```python
from build123d import *

# Parameters (mm, degrees)
BOSS_EXTRUDE4_DEPTH = 10
SKETCH4_R           = 5
CUT_EXTRUDE2_DEPTH  = 10
BOSS_EXTRUDE5_DEPTH = 40
SKETCH6_R           = 5
CUT_EXTRUDE4_DEPTH  = 60
SKETCH7_W           = 45
SKETCH7_H           = 20
CUT_EXTRUDE5_DEPTH  = 40
RIB1_REACH          = 78.889
SKETCH8_WALL_W      = 212.346557286
SKETCH8_WALL_H      = 6
SKETCH9_R           = 20
BOSS_EXTRUDE7_DEPTH = 25
BOSS_EXTRUDE7_TAPER = 21.8
SKETCH15_R          = 5
CUT_EXTRUDE6_DEPTH  = 25


with BuildPart() as part:
    # Sketch1 → Boss-Extrude4 (new body)
    with BuildSketch(Plane(origin=(0, 0, 0), x_dir=(1, 0, 0), z_dir=(0, 1, 0))):
        with BuildLine():
            Line((-35.119052847, -30), (35.119052847, -30))
            ThreePointArc((35.119052847, -30), (45.725654565, -25.606601718), (50.119052847, -15))
            Line((50.119052847, -15), (50.119052847, 15))
            ThreePointArc((50.119052847, 15), (45.725654565, 25.606601718), (35.119052847, 30))
            Line((35.119052847, 30), (-35.119052847, 30))
            ThreePointArc((-35.119052847, 30), (-45.725654565, 25.606601718), (-50.119052847, 15))
            Line((-50.119052847, 15), (-50.119052847, -15))
            ThreePointArc((-50.119052847, -15), (-45.725654565, -25.606601718), (-35.119052847, -30))
        make_face()
    extrude(amount=BOSS_EXTRUDE4_DEPTH)

    # Sketch4 → Cut-Extrude2 (cut)
    with BuildSketch(Plane(origin=(0, 10, 0), x_dir=(1, 0, 0), z_dir=(0, 1, 0))):
        with Locations(Location((-35.054653665, 15.038511516, 0), (0, 0, 270))):
            Circle(SKETCH4_R)
        with Locations(Location((-35.054653665, -15.038511516, 0), (0, 0, 90))):
            Circle(SKETCH4_R)
    extrude(amount=-CUT_EXTRUDE2_DEPTH, mode=Mode.SUBTRACT)

    # Sketch5 → Boss-Extrude5 (add)
    with BuildSketch(Plane(origin=(0, 10, 0), x_dir=(1, 0, 0), z_dir=(0, 1, 0))):
        with BuildLine():
            Line((-10.119052847, -20), (-10.119052847, 20))
            Line((-10.119052847, 20), (29.880947153, 20))
            ThreePointArc((29.880947153, 20), (49.880947153, 0), (29.880947153, -20))
            Line((29.880947153, -20), (-10.119052847, -20))
        make_face()
    extrude(amount=BOSS_EXTRUDE5_DEPTH)

    # Sketch6 → Cut-Extrude4 (cut)
    with BuildSketch(Plane(origin=(0, 50, 0), x_dir=(1, 0, 0), z_dir=(0, 1, 0))):
        with Locations(Location((29.880947153, 0, 0), (0, 0, 270))):
            Circle(SKETCH6_R)
    extrude(amount=-CUT_EXTRUDE4_DEPTH, mode=Mode.SUBTRACT)

    # Sketch7 → Cut-Extrude5 (cut)
    with BuildSketch(Plane.XY.offset(20)):
        with Locations((27.380947153, 30)):
            Rectangle(SKETCH7_W, SKETCH7_H)
    extrude(amount=-CUT_EXTRUDE5_DEPTH, mode=Mode.SUBTRACT)

    # Sketch8 wall → Rib1 (add, up to next)
    with BuildSketch(Plane(origin=(-30.119052847, 30, 0), x_dir=(0.707106781187, 0.707106781187, 0), z_dir=(-0.707106781187, 0.707106781187, 0)), mode=Mode.PRIVATE) as rib1_sk1:
        Rectangle(SKETCH8_WALL_W, SKETCH8_WALL_H)
    rib1_tool1 = extrude(rib1_sk1.sketch, amount=-RIB1_REACH, mode=Mode.PRIVATE) - part.part
    add(rib1_tool1.solids().sort_by_distance((-30.119052847, 30, 0))[0])

    # Sketch9 → Boss-Extrude7 (add)
    with BuildSketch(Plane(origin=(0, 50, 0), x_dir=(1, 0, 0), z_dir=(0, 1, 0))):
        with Locations((29.880947153, 0)):
            Circle(SKETCH9_R)
    extrude(amount=BOSS_EXTRUDE7_DEPTH, taper=BOSS_EXTRUDE7_TAPER)

    # Sketch15 → Cut-Extrude6 (cut)
    with BuildSketch(Plane(origin=(0, 75, 0), x_dir=(1, 0, 0), z_dir=(0, 1, 0))):
        with Locations(Location((29.9308784, 0, 0), (0, 0, 270))):
            Circle(SKETCH15_R)
    extrude(amount=-CUT_EXTRUDE6_DEPTH, mode=Mode.SUBTRACT)


solid = part.part
```
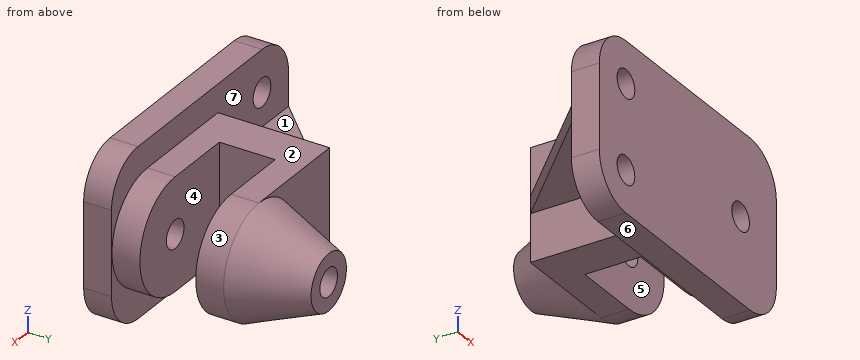
Input: part model. Units: mm. Frame: model coordinates. Face numbers are marked on the shaded views. A direction names the side the tool comes from. Coordinates: 2 decimals unless noted, no trailing zeros. Write each loop counter-clockwise with the first axis right and the second up, starting at its lowest first coordinate (ties: lowest second). Pieces come first, ordered by that corner, then holes.
1) Set-up query: the marked faces 1, 2, 3 and 4. Return all of +Z, -Z, +X, -X, +Y, -Y with unobstructed straight access to the full face (end or side cutting, diameter ignored); none if empty.
2) Section A-A on y = 41.5. Output: boundary loops of the cut face in (x, z).
3) Section B-B on x = -7. Output: boundary loops of the cut face in (y, z), and give its area (3 significant figures).
4) Section D-D on y = 26.5. Output: boundary loops of the cut face in (x, z), and give its area (3 significant figures).
5) Material intervals for line 1 along Y through (x, z) = (18.5, -16.5); line 2 along Y through (x, z) = (-19.5, -26.5); line 3 along Z through (x, y) = (6.5, 47), sorted ascending.
6) Pin query (flat end, axial travel): pin 1 Ø8.5 at (y, z) = (25.5, 14) entering from -X; pin 2 Ø5 at (x, y) = (27, 43) entering from -Z; pin 3 Ø3 at (x, z) = (-2.5, -9) entering from +Y. Return the tip coordinate at first contact, or that it passes through.
7) Mould query, pull axis Y, two halves, no side actions, for the marked faces 5, 6 and 7. Classes: pulls with the +Y half, pulls with the -Y half, needs draft (parallel to the pull), parting line crosses it, or undercut.
8) Section C-C on z = 0. State how many separate pieces and enclosed holes the cut face has, and give its area (3 significant figures).
Check result:
1. face 1: +Z, -X, +Y
1. face 2: +Z, +X, -X, +Y
1. face 3: +X, +Y
1. face 4: +Z, -Z, +X
2. outline: (-18.62, -3) - (-10.12, -3) - (-10.12, -20) - (29.88, -20) arc R20 ccw to (29.88, 20) - (-10.12, 20) - (-10.12, 3) - (-18.62, 3) - close; hole circle Ø10 at (29.88, 0)
3. outline: (0, -30) - (10, -30) - (10, -20) - (50, -20) - (50, 20) - (10, 20) - (10, 30) - (0, 30) - close
3. area: 2,200 mm2
4. outline: (-33.62, -3) - (-10.12, -3) - (-10.12, -20) - (4.88, -20) - (4.88, 20) - (-10.12, 20) - (-10.12, 3) - (-33.62, 3) - close
4. area: 741 mm2
5. line 1: y = 0 to 20, 40 to 50
5. line 2: y = 0 to 10
5. line 3: z = -20 to 20
6. pin 1: stops at x = -10.12
6. pin 2: stops at z = -20
6. pin 3: stops at y = 50
7. face 5: undercut
7. face 6: needs draft
7. face 7: pulls with the +Y half
8. separate pieces: 3
8. enclosed holes: 0
8. area: 3,500 mm2
